Build history of the part. All positions in model axes, mm. A direction names the side the tool comes from. Round coordinates to 2 decimals unless told otherwise and drop trailing zeros. Write each loop counter-clockwise with the first axis right and the second up, starting at its lowest first coordinate (ties: lowest second). Pieces come first, ordered by that corner, then holes. Notation, with made-up numbers: M 8,8 L 19,8 A16 cw 19,20 Z; hole C 60.5,16.5 d8. An arc over 180 degrees is marked long. One line per item, written item: value. Start each with the question number.
```python
from build123d import *

# Parameters (mm, degrees)
F1_DEPTH = 38.1
F2_R     = 1.016
F3_R     = 1.016
F4_R     = 0.508
F5_R     = 0.508


with BuildPart() as f1:
    # F0 (on Front) → F1 (new body)
    with BuildSketch(Plane.XZ):
        Polygon((-4.299126, 0.79375), (-4.299126, -0.79375), (4.299126, -0.79375), (4.299126, 0.79375), (1.476904, 0.79375), (1.476904, 0), (3.964072, 0.321753), (3.964072, -0.412909), (-3.964072, -0.412909), (-3.964072, 0.321753), (-1.476904, 0), (-1.476904, 0.79375), align=None)
    extrude(amount=F1_DEPTH)

    # F2
    f2_edges = [f1.edges().sort_by_distance(p)[0] for p in [
        (-4.299126, -19.05, 0.79375),
    ]]
    fillet(f2_edges, radius=F2_R)

    # F3
    f3_edges = [f1.edges().sort_by_distance(p)[0] for p in [
        (4.299126, -19.05, 0.79375),
    ]]
    fillet(f3_edges, radius=F3_R)

    # F4
    f4_edges = [f1.edges().sort_by_distance(p)[0] for p in [
        (-1.476904, -19.05, 0.79375),
    ]]
    fillet(f4_edges, radius=F4_R)

    # F5
    f5_edges = [f1.edges().sort_by_distance(p)[0] for p in [
        (1.476904, -19.05, 0.79375),
    ]]
    fillet(f5_edges, radius=F5_R)


solid = f1.part
```
Item 1: Cut at C-C, the plane x = -0.75. Write the cut outline in (y, z), plus the area to 3 significant figures.
Item 2: Cut at A-A, the plane y = -16.5. Write the cut outline in (x, z), plus the area to 3 significant figures.
Item 3: Drill centre lines: line 1 (X direction, y = -18.5, z = -0.2); line 2 (Z direction, x = 2.25, y = -22.5); line 3 (Z direction, x = 1, y = -9.5). Where is each one in solid material? Low to high.
Item 4: Two-plate mould, pull along Z, no slides. Class faces 1 (the flat face through (3, -19, 0.794)), 2 (the flat face through (0, -19, -0.794)), 3 (the flat face through (2.7, -18.78, 0.16)): pulls with the +Z half, pulls with the -Z half, needs draft (parallel to the pull), parting line crosses it, or undercut.
Item 5: Cut at B-B, the plane x = 2.75. Write the cut outline in (y, z), plus the area to 3 significant figures.
Item 6: Which spindle directions (+Z, -Z, +X, -X, +Y, -Y) get a long thin tool onto all of the face, cutting with end or side? Do faces 4 (the flat face through (0, -19, -0.413)), 5 (the cylindrical face through (4, -19.3, 0.5)). Say none if no direction does.
Computed values:
1. outline: M -38.1,-0.79 L 0,-0.79 L 0,-0.41 L -38.1,-0.41 Z
1. area: 14.5 mm2
2. outline: M -4.3,-0.79 L 4.3,-0.79 L 4.3,-0.22 A1.02 ccw 3.28,0.79 L 1.98,0.79 A0.51 ccw 1.48,0.29 L 1.48,0 L 3.96,0.32 L 3.96,-0.41 L -3.96,-0.41 L -3.96,0.32 L -1.48,0 L -1.48,0.29 A0.51 ccw -1.98,0.79 L -3.28,0.79 A1.02 ccw -4.3,-0.22 Z
2. area: 6.68 mm2
3. line 1: x = -4.3 to -3.96, 3.96 to 4.3
3. line 2: z = -0.79 to -0.41, 0.1 to 0.79
3. line 3: z = -0.79 to -0.41
4. face 1: pulls with the +Z half
4. face 2: pulls with the -Z half
4. face 3: undercut
5. outline: M -38.1,-0.79 L 0,-0.79 L 0,-0.41 L -38.1,-0.41 Z; M -38.1,0.16 L 0,0.16 L 0,0.79 L -38.1,0.79 Z
5. area: 38.5 mm2
6. face 4: +Y, -Y
6. face 5: +Z, +X, +Y, -Y
